from build123d import *
from build123d.topology import SkipClean

# Parameters (mm, degrees)
SKETCH1_R           = 43
BOSS_EXTRUDE1_DEPTH = 2
SKETCH2_R           = 43
SKETCH2_R_2         = 41
BOSS_EXTRUDE2_DEPTH = 20
BOSS_EXTRUDE3_DEPTH = 100
SKETCH4_R           = 43
SKETCH4_R_2         = 41
BOSS_EXTRUDE4_DEPTH = 20
BOSS_EXTRUDE5_DEPTH = 5
BOSS_EXTRUDE6_DEPTH = 127
SKETCH7_W           = 7.682690019
SKETCH7_H           = 127
BOSS_EXTRUDE7_DEPTH = 5
SKETCH10_R          = 2
CUT_EXTRUDE2_DEPTH  = 15


with BuildPart() as part:
    # Sketch1 → Boss-Extrude1 (new body)
    with BuildSketch(Plane.XY):
        Circle(SKETCH1_R)
    extrude(amount=BOSS_EXTRUDE1_DEPTH)

    # Sketch2 → Boss-Extrude2 (add)
    with BuildSketch(Plane.XY.offset(2)):
        Circle(SKETCH2_R)
        Circle(SKETCH2_R_2, mode=Mode.SUBTRACT)
    extrude(amount=BOSS_EXTRUDE2_DEPTH)

    # Sketch3 → Boss-Extrude3 (add)
    with SkipClean():  # the faces are left unmerged after this step: merging them gives an invalid solid
        with BuildSketch(Plane.XY.offset(22)):
            with BuildLine():
                Line((39.761790704, 10), (41.821047333, 10))
                ThreePointArc((41.821047333, 10), (43, 0), (41.821047333, -10))
                Line((41.821047333, -10), (39.761790704, -10))
                ThreePointArc((39.761790704, -10), (41, 0), (39.761790704, 10))
            make_face()
            with BuildLine():
                Line((-41.821047333, -10), (-39.761790704, -10))
                ThreePointArc((-39.761790704, -10), (-41, 0), (-39.761790704, 10))
                Line((-39.761790704, 10), (-41.821047333, 10))
                ThreePointArc((-41.821047333, 10), (-43, 0), (-41.821047333, -10))
            make_face()
        extrude(amount=BOSS_EXTRUDE3_DEPTH)

    # Sketch4 → Boss-Extrude4 (add)
    with SkipClean():  # the faces are left unmerged after this step: merging them gives an invalid solid
        with BuildSketch(Plane.XY.offset(122)):
            Circle(SKETCH4_R)
            Circle(SKETCH4_R_2, mode=Mode.SUBTRACT)
        extrude(amount=BOSS_EXTRUDE4_DEPTH)

    # Sketch5 → Boss-Extrude5 (add)
    with SkipClean():  # the faces are left unmerged after this step: merging them gives an invalid solid
        with BuildSketch(Plane.XY.offset(142)):
            with BuildLine():
                ThreePointArc((-4.6225, 42.750818633), (-6.633671033, 51.082901463), (-9, 59.3211598))
                ThreePointArc((-9, 59.3211598), (-60, 0), (-9, -59.3211598))
                ThreePointArc((-9, -59.3211598), (-6.633671033, -51.082901463), (-4.6225, -42.750818633))
                ThreePointArc((-4.6225, -42.750818633), (-43, 0), (-4.6225, 42.750818633))
            make_face()
        boss_extrude5 = extrude(amount=-BOSS_EXTRUDE5_DEPTH)

    # Mirror1: Boss-Extrude5 across plane
    with SkipClean():  # the faces are left unmerged after this step: merging them gives an invalid solid
        add(boss_extrude5.mirror(Plane(origin=(0, 0, 134.5), x_dir=(1, 0, 0), z_dir=(0, 0, -1))))

    # Sketch6 → Boss-Extrude6 (add)
    with SkipClean():  # the faces are left unmerged after this step: merging them gives an invalid solid
        with BuildSketch(Plane(origin=(0, 0, 127), x_dir=(-1, 0, 0), z_dir=(0, 0, -1))):
            with BuildLine():
                ThreePointArc((43, 0), (42.704244726, -5.034628323), (41.821047333, -10))
                Line((41.821047333, -10), (59.160797831, -10))
                ThreePointArc((59.160797831, -10), (59.789831367, -5.017575617), (60, 0))
                ThreePointArc((60, 0), (59.789831367, 5.017575617), (59.160797831, 10))
                Line((59.160797831, 10), (41.821047333, 10))
                ThreePointArc((41.821047333, 10), (42.704244726, 5.034628323), (43, 0))
            make_face()
            with BuildLine():
                ThreePointArc((60, 0), (59.789831367, -5.017575617), (59.160797831, -10))
                Line((59.160797831, -10), (80, -10))
                Line((80, -10), (80, 10))
                Line((80, 10), (59.160797831, 10))
                ThreePointArc((59.160797831, 10), (59.789831367, 5.017575617), (60, 0))
            make_face()
        extrude(amount=BOSS_EXTRUDE6_DEPTH)

    # Sketch7 → Cut-Revolve1 (revolve, cut)
    with SkipClean():  # the faces are left unmerged after this step: merging them gives an invalid solid
        with BuildSketch(Plane(origin=(0, 0, 0), x_dir=(1, 0, 0), z_dir=(0, 1, 0)), mode=Mode.PRIVATE) as cut_revolve1_sk:
            with Locations((-83.84134501, -63.5)):
                Rectangle(SKETCH7_W, SKETCH7_H)
            Polygon((-80, 0), (-80, -127), (-43, 0), align=None)
        revolve(cut_revolve1_sk.sketch.rotate(Axis((0, 0, -46.383399508), (0, 0, 1)), 276.171221478), axis=Axis((0, 0, -46.383399508), (0, 0, 1)), mode=Mode.SUBTRACT)

    # Sketch8 → Boss-Extrude7 (add)
    with SkipClean():  # the faces are left unmerged after this step: merging them gives an invalid solid
        with BuildSketch(Plane.XY.offset(127)):
            with BuildLine():
                Line((-59.160797831, 10), (-79.372539332, 10))
                ThreePointArc((-79.372539332, 10), (-80, 0), (-79.372539332, -10))
                Line((-79.372539332, -10), (-59.160797831, -10))
                ThreePointArc((-59.160797831, -10), (-60, 0), (-59.160797831, 10))
            make_face()
        extrude(amount=BOSS_EXTRUDE7_DEPTH)

    # Sketch10 → Cut-Extrude2 (cut)
    with SkipClean():  # the faces are left unmerged after this step: merging them gives an invalid solid
        with BuildSketch(Plane.XY.offset(142)):
            with Locations((-13.1997713, 49.262217141)):
                Circle(SKETCH10_R)
            with Locations((-13.1997713, -49.262217141)):
                Circle(SKETCH10_R)
        extrude(amount=-CUT_EXTRUDE2_DEPTH, mode=Mode.SUBTRACT)


solid = part.part
Work out the finished part from the listing and answer in its coordinate system (mm). A direction names the side the tool comes from. Give positions to 0.01 mm unless a question says otherwise; leave off trailing zeros. Order: outer loops, then holes, each group sorted by start corner. A loop starts at its lowest first (then second) coordinate and runs counter-clockwise, first axis right, second up. Notation, with made-up numbers: (-0.5, -31.75) -> (30.5, -31.75) arc R17 cw to (30.5, -4.75) -> close; hole circle Ø10 at (3, 82). An arc over 180 degrees is marked (long way). One line per item, written item: value.
Item 1: Flat-ended cylindrical pins translate along their axes: P1, Ø16, axis at x = -72.5, y = 2.5, coming from the +Z side; P2, Ø6, axis at y = -2, z = 15.5, coming from the -X side; P3, Ø16.5, axis at x = -10.5, y = 34, coming from the +Z side; P4, Ø1.6, axis at x = -41, z = 95, coming from the -Y side. Find the tip coordinate at first contact, or state that the pin passes through.
Answer sheet:
P1: z = 132
P2: x = -48.36
P3: z = 142
P4: y = -10
Item 2: Determine the mould class of faces 6 (the flat face through (-45, 1, 137)), 7 (the cylindrical face through (-59.99, 1.19, 139.54)), 8 (the flat face through (-32, -34, 127)), 9 (the flat face through (-0.2, 41.2, 122)) for opening direction Z: released by +Z, released by -Z, zero draft, split by the parting line, or undercut.
Answer sheet:
face 6: undercut
face 7: zero draft
face 8: released by -Z
face 9: undercut
Item 3: Find section C-C, the plane z = 12. Give the vertices of the cut face in (x, y).
Answer sheet:
outline: (-45.41, -10) -> (-41.82, -10) arc R43 ccw (long way) to (-41.82, 10) -> (-45.41, 10) arc R46.5 ccw to start; hole circle Ø82 at (0, 0)
Item 4: Straight lines are drawn through the part: probe 1 along Z at (x, y) = (-14.5, -41); probe 2 along X at (y, z) = (0, 129); probe 3 along Y at (x, z) = (0, 11). For each, find the intervals that lie inside material, in ascending order.
Answer sheet:
probe 1: 127 to 132, 137 to 142
probe 2: -80 to -41, 41 to 43
probe 3: -43 to -41, 41 to 43
Item 5: Find section A-A, the plane x = 0. Give the vertices of the cut face in (y, z), plus the area to 3 significant figures.
Answer sheet:
outline: (-43, 0) -> (43, 0) -> (43, 22) -> (41, 22) -> (41, 2) -> (-41, 2) -> (-41, 22) -> (-43, 22) -> close; (-43, 122) -> (-41, 122) -> (-41, 142) -> (-43, 142) -> close; (41, 122) -> (43, 122) -> (43, 142) -> (41, 142) -> close
area: 332 mm²
Item 6: A tool of negligible diameter and unlimited length cuts with its end or side. For faces 1 (the flat face through (-32, 35, 127)), 2 (the cylindrical face through (-12.125, 50.949, 139.535)), 3 (the flat face through (-0.2, 41.2, 22)), 4 (the flat face through (-1, 1, 2)), 5 (the cylindrical face through (-42.44, -42.41, 129.46)), from which of +Z, -Z, +X, -X, +Y, -Y can it reach the whole face along a straight path? Write none if from no direction.
Answer sheet:
face 1: -Z, -X, +Y
face 2: +Z, -Z
face 3: +X, -X, +Y
face 4: +Z
face 5: +Z, -Z, -X, -Y
Item 7: Find section B-B, the plane z = 40. Give the vertices of the cut face in (x, y), plus the area to 3 significant figures.
Answer sheet:
outline: (-53.73, -10) -> (-39.76, -10) arc R41 cw to (-39.76, 10) -> (-53.73, 10) arc R54.65 ccw to start; (39.76, -10) -> (41.82, -10) arc R43 ccw to (41.82, 10) -> (39.76, 10) arc R41 cw to start
area: 316 mm²
Item 8: Find section D-D, the plane x = -17.5. Give the vertices of the cut face in (y, z), plus the area to 3 significant figures.
Answer sheet:
outline: (-57.39, 127) -> (-39.28, 127) -> (-39.28, 122) -> (-37.08, 122) -> (-37.08, 142) -> (-57.39, 142) -> (-57.39, 137) -> (-39.28, 137) -> (-39.28, 132) -> (-57.39, 132) -> close; (-39.28, 0) -> (39.28, 0) -> (39.28, 22) -> (37.08, 22) -> (37.08, 2) -> (-37.08, 2) -> (-37.08, 22) -> (-39.28, 22) -> close; (37.08, 122) -> (39.28, 122) -> (39.28, 127) -> (57.39, 127) -> (57.39, 132) -> (39.28, 132) -> (39.28, 137) -> (57.39, 137) -> (57.39, 142) -> (37.08, 142) -> close
area: 695 mm²
